```python
from build123d import *

# Parameters (mm, degrees)
SKETCH1_W                     = 100
SKETCH1_H                     = 100
BOSS_EXTRUDE1_DEPTH           = 1.7
SKETCH2_W                     = 30.2
SKETCH2_H                     = 9
SKETCH2_W_2                   = 20
BOSS_EXTRUDE2_DEPTH           = 13
SKETCH3_W                     = 49
SKETCH3_H                     = 29
BOSS_EXTRUDE3_DEPTH           = 5
SKETCH4_W                     = 19.36
SKETCH4_H                     = 8.32
BOSS_EXTRUDE4_DEPTH           = 4.13
SKETCH5_W                     = 54.5
SKETCH5_H                     = 33
BOSS_EXTRUDE5_DEPTH           = 12.5
M3_CLEARANCE_HOLE1_AT_2_COUNT = 2
M3_CLEARANCE_HOLE1_AT_2_PITCH = 48


with BuildPart() as part:
    # Sketch1 → Boss-Extrude1 (new body)
    with BuildSketch(Plane(origin=(0, 0, 0), x_dir=(1, 0, 0), z_dir=(0, 1, 0))):
        Rectangle(SKETCH1_W, SKETCH1_H)
    extrude(amount=BOSS_EXTRUDE1_DEPTH)

    # Sketch2 → Boss-Extrude2 (add)
    with BuildSketch(Plane(origin=(0, 1.7, 0), x_dir=(1, 0, 0), z_dir=(0, 1, 0))):
        with Locations((22.4, 45.5)):
            Rectangle(SKETCH2_W, SKETCH2_H)
        with Locations((-33, 45.5)):
            Rectangle(SKETCH2_W_2, SKETCH2_H)
    extrude(amount=BOSS_EXTRUDE2_DEPTH)

    # Sketch3 → Boss-Extrude3 (add)
    with BuildSketch(Plane(origin=(0, 1.7, 0), x_dir=(1, 0, 0), z_dir=(0, 1, 0))):
        with Locations((-25.5, 18)):
            Rectangle(SKETCH3_W, SKETCH3_H)
    extrude(amount=BOSS_EXTRUDE3_DEPTH)

    # Sketch4 → Boss-Extrude4 (add)
    with BuildSketch(Plane(origin=(0, 1.7, 0), x_dir=(1, 0, 0), z_dir=(0, 1, 0))):
        with Locations((29.02, 21.32)):
            Rectangle(SKETCH4_W, SKETCH4_H)
        with Locations((29.02, -6.7)):
            Rectangle(SKETCH4_W, SKETCH4_H)
        with Locations((29.02, -34.72)):
            Rectangle(SKETCH4_W, SKETCH4_H)
    extrude(amount=BOSS_EXTRUDE4_DEPTH)

    # Sketch5 → Boss-Extrude5 (add)
    with BuildSketch(Plane(origin=(0, 1.7, 0), x_dir=(1, 0, 0), z_dir=(0, 1, 0))):
        with Locations((-17.75, -28.3)):
            Rectangle(SKETCH5_W, SKETCH5_H)
    extrude(amount=BOSS_EXTRUDE5_DEPTH)

    # Sketch9 → M3 Clearance Hole1 (revolve, cut)
    with BuildSketch(Plane(origin=(-37, 1.7, 4.15), x_dir=(0, 0, 1), z_dir=(1, 0, 0))):
        Polygon((0, 0), (0, 1.7), (1.7, 1.7), (1.7, 0.025), (1.725, 0), align=None)
    m3_clearance_hole1 = revolve(axis=Axis((-37, 8.05, 4.15), (0, -1, 0)), mode=Mode.SUBTRACT)

    # M3 Clearance Hole1 at 2: M3 Clearance Hole1 ×2
    with Locations(*[(i * M3_CLEARANCE_HOLE1_AT_2_PITCH, 0, 0) for i in range(1, M3_CLEARANCE_HOLE1_AT_2_COUNT)]):
        add(m3_clearance_hole1, mode=Mode.SUBTRACT)


solid = part.part
```
Input: part model. Units: mm. Frame: model coordinates. A direction names the side the tool comes from. Coordinates: 2 decimals unless noted, no trailing zeros. Loops run counter-clockwise (first coordinate to the right, second up) from the corner with the lowest first, then second, coordinate; pieces in that order, holes last. Notation, with made-up numbers: M -34,12 L -6,12 A17 ccw -6,42 Z; hole C 86,36.5 d7. An arc over 180 degrees is marked long. One line per item, written item: value.
(1) Section A-A (x = -37). Output: boundary loops of the cut face in (y, z) (3 decimals).
Filled in:
outline: M 0,-50 L 14.7,-50 L 14.7,-41 L 1.7,-41 L 1.7,-32.5 L 6.7,-32.5 L 6.7,-3.5 L 1.7,-3.5 L 1.7,2.425 L 1.675,2.45 L 0,2.45 Z; M 0,5.85 L 1.675,5.85 L 1.7,5.875 L 1.7,11.8 L 14.2,11.8 L 14.2,44.8 L 1.7,44.8 L 1.7,50 L 0,50 Z
(2) Line query: line 1 along X through (y, z) = (1.25, 4.15); line 2 along X through (y, z) = (5.25, -44); line 3 along Z through (x, y) = (11, 0.75). Output: solid intervals per line, ascending. Write a range as from..to.
Filled in:
line 1: -50..-38.7, -35.3..9.3, 12.7..50
line 2: -43..-23, 7.3..37.5
line 3: -50..2.45, 5.85..50
(3) Section C-C (y = 9). Output: boundary loops of the cut face in (x, z), and give its area (3 significant figures).
Filled in:
outline: M -45,11.8 L 9.5,11.8 L 9.5,44.8 L -45,44.8 Z; M -43,-50 L -23,-50 L -23,-41 L -43,-41 Z; M 7.3,-50 L 37.5,-50 L 37.5,-41 L 7.3,-41 Z
area: 2,250 mm^2
(4) Pull-direction query (Z, two-part tool) for faces 1 (the flat face through (-50, 2, -10)), 2 (the cylindrical face through (12.03, 0.85, 2.8)), 3 (the flat face through (29, 4, 38.88)); classes: +Z half, -Z half, draft (parallel to the pull), parting line (faces both ways), or undercut.
Filled in:
face 1: draft
face 2: undercut
face 3: +Z half
(5) Pin query (flat end, axial travel): pin 1 (1 mm diameter, centred on x = 8.5, y = 11, fed in from +Z); pin 2 (1.5 mm diameter, centred on y = 3.5, z = 20, fed in from -X); pin 3 (8 mm diameter, centred on x = 32.5, y = 12.5, fed in from +Z). Return the tip coordinate at first contact, or that it passes through.
Filled in:
pin 1: z = 44.8
pin 2: x = -45
pin 3: z = -41
(6) Section B-B (z = 4.15). Output: boundary loops of the cut face in (x, y) (3 decimals), and give its area (3 significant figures).
Filled in:
outline: M -50,0 L -38.7,0 L -38.7,1.675 L -38.725,1.7 L -50,1.7 Z; M -35.3,0 L 9.3,0 L 9.3,1.675 L 9.275,1.7 L -35.275,1.7 L -35.3,1.675 Z; M 12.7,0 L 50,0 L 50,1.7 L 38.7,1.7 L 38.7,5.83 L 19.34,5.83 L 19.34,1.7 L 12.725,1.7 L 12.7,1.675 Z
area: 238 mm^2
(7) Reachability of faces 4 (the flat face through (-18, 8, 44.8)), 5 (the flat face through (19.34, 4, -21)), 6 (the flat face through (38.7, 4, 35)), 7 (the flat face through (19.34, 4, 7)), 8 (the flat face through (29, 5.83, -21)) from +Z, -Z, +X, -X, +Y, -Y: full face, straight path, thin tool, end or side. Return the list, or none.
Filled in:
face 4: +Z, +X, -X, +Y
face 5: +Z, +Y
face 6: +Z, -Z, +X, +Y
face 7: +Z, -X, +Y
face 8: +Z, +X, +Y
(8) Section D-D (x = 3). Output: boundary loops of the cut face in (y, z), and give its area (4 significant figures).
Filled in:
outline: M 0,-50 L 1.7,-50 L 1.7,11.8 L 14.2,11.8 L 14.2,44.8 L 1.7,44.8 L 1.7,50 L 0,50 Z
area: 582.5 mm^2
